Geometry: final body of the model. Coordinates: model frame, mm. A direction names the side the tool comes from. Round coordinates to 2 decimals unless told otherwise and drop trailing zeros. Loops run counter-clockwise (first coordinate to the right, second up) from the corner with the lowest first, then second, coordinate; pieces in that order, holes last. Notation, with made-up numbers: (-3, 50) - (14, 50) arc R11 cw to (14, 65) - close; hole circle Ø1 at (14, 39.25). An arc over 180 degrees is marked (long way). Return JSON: item names as keys, results as strings. Group by question number.
1. Section C-C on y = 20. Return loops of the section in (x, z) (3 decimals), and give its area (3 significant figures).
2. Section D-D on x = 88. Return loops of the section in (y, z) (3 decimals).
3. Section B-B on y = -39. Return loops of the section in (x, z) (3 decimals), and give its area (3 significant figures).
4. First-contact query: pin 1 Ø4 at (x, z) = (32, 19) entering from +Y; pin 2 Ø8 at (y, z) = (-10, 40) entering from +X; pin 3 Ø12 at (y, z) = (1, 50.5) entering from +X (3 decimals); pin 4 Ø15 at (y, z) = (-22.5, 19.5) entering from +X (3 decimals). Flat tips, straight axial feed; report the tip coordinate or a pass-through.
5. Material intervals for probe 1 along Y at (x, z) = (11, 39) (3 decimals); probe 2 along Z at (x, y) = (-19.5, 52) (3 decimals); probe 3 along X at (y, z) = (-22, 13) (3 decimals), sorted ascending.
6. Set-up query: faces 1 (the face through (32.73, -20.7, 51.97)), 2 (the face through (9, 0, 31)), 3 (the face through (45.8, -0.4, 38.1)), 4 (the face through (86, 0, 38.1)), 5 (the face through (47, -25.4, 42)). Return all of +Z, -Z, +X, -X, +Y, -Y with unobstructed straight access to the full face (end or side cutting, diameter ignored); none if empty.
7. Section A-A on z = 0. Return loops of the section in (x, y) (3 decimals).
from build123d import *

# Parameters (mm, degrees)
F1_DEPTH = 63.5
F0_W     = 25.7705491662
F0_H     = 19.05
F2_DEPTH = 25.4
F3_DEPTH = 15.875
F4_DEPTH = 25.4
F6_R     = 6.35


with BuildPart() as f1:
    # F0 (on Front) → F1 (new body, symmetric)
    with BuildSketch(Plane.XZ):
        Polygon((22.225, 9.525), (-41.275, 9.525), (-41.275, -9.525), (41.275, -9.525), (41.275, 9.525), align=None)
    extrude(amount=F1_DEPTH, both=True)

    # F0 (on Front) → F2 (join, symmetric)
    with BuildSketch(Plane.XZ):
        with BuildLine():
            Line((22.225, 27.0002), (22.225, 9.525))
            Line((22.225, 9.525), (41.275, 9.525))
            Line((41.275, 9.525), (41.275, 27.0002))
            ThreePointArc((41.275, 27.0002), (45.9246798487, 38.2255201513), (57.15, 42.8752))
            Line((57.15, 42.8752), (60.325, 42.8752))
            Line((60.325, 42.8752), (60.325, 61.9252))
            Line((60.325, 61.9252), (57.15, 61.9252))
            ThreePointArc((57.15, 61.9252), (32.4542956671, 51.6959043329), (22.225, 27.0002))
        make_face()
        with Locations((73.2102745831, 52.4002)):
            Rectangle(F0_W, F0_H)
    extrude(amount=F2_DEPTH, both=True)

    # F0 (on Front) → F3 (join)
    with BuildSketch(Plane.XZ):
        with BuildLine():
            add(Edge.make_bspline(
                [(-41.275, 9.525), (-11.6340629756, 43.7753386796), (15.0888795033, 63.8811737299), (57.15, 61.9252)],
                knots=[0, 0, 0, 0, 111.5045361635, 111.5045361635, 111.5045361635, 111.5045361635], degree=3))
            Line((-41.275, 9.525), (22.225, 9.525))
            Line((22.225, 9.525), (22.225, 27.0002))
            ThreePointArc((22.225, 27.0002), (32.4542956671, 51.6959043329), (57.15, 61.9252))
        make_face()
    extrude(amount=F3_DEPTH)

    # F0 (on Front) → F4 (join, symmetric)
    with BuildSketch(Plane.XZ):
        with Locations((73.2102745831, 52.4002)):
            Rectangle(F0_W, F0_H)
    extrude(amount=F4_DEPTH, both=True)

    # F0 (on Front) → F5 (revolve)
    with BuildSketch(Plane.XZ):
        Polygon((86.0955491662, 66.675), (86.0955491662, 61.9252), (86.0955491662, 42.8752), (86.0955491662, 38.1), (111.125, 38.1), (111.125, 66.675), align=None)
    revolve(axis=Axis((86.0955491662, 0, 52.3875), (0, 0, -1)))

    # F6
    f6_edges = [f1.edges().sort_by_distance(p)[0] for p in [
        (41.275, -63.5, 0),
        (-41.275, -63.5, 0),
        (-41.275, 0, -9.525),
        (0, 63.5, -9.525),
        (41.275, 0, -9.525),
        (0, -63.5, -9.525),
        (-41.275, 63.5, 0),
        (41.275, 63.5, 0),
    ]]
    fillet(f6_edges, radius=F6_R)


solid = f1.part
Taken from the geometry:
{
 "1": {"outline": "(-41.275, -3.175) arc R6.35 ccw to (-34.925, -9.525) - (34.925, -9.525) arc R6.35 ccw to (41.275, -3.175) - (41.275, 27) arc R15.875 cw to (57.15, 42.875) - (71.047, 42.875) - (71.047, 38.1) - (101.145, 38.1) - (101.145, 66.675) - (71.047, 66.675) - (71.047, 61.925) - (57.15, 61.925) arc R34.925 ccw to (22.225, 27) - (22.225, 9.525) - (-41.275, 9.525) - close", "area": "3,770 mm2"},
 "2": {"outline": "(-24.957, 38.1) - (24.957, 38.1) - (24.957, 66.675) - (-24.957, 66.675) - close"},
 "3": {"outline": "(-41.275, -3.175) arc R6.35 ccw to (-34.925, -9.525) - (34.925, -9.525) arc R6.35 ccw to (41.275, -3.175) - (41.275, 9.525) - (-41.275, 9.525) - close", "area": "1,560 mm2"},
 "4": {"pin 1": "y = 25.4", "pin 2": "x = 110.4", "pin 3": "x = 111.125", "pin 4": "x = 41.275"},
 "5": {"probe 1": "-15.875 to 0", "probe 2": "-9.525 to 9.525", "probe 3": "22.225 to 41.275"},
 "6": {"face 1": "+Z, -X, -Y", "face 2": "+Z, -X, +Y", "face 3": "-Z, +Y, -Y", "face 4": "-Z, +X, +Y, -Y", "face 5": "+Z, +X, -X, -Y"},
 "7": {"outline": "(-41.275, -57.15) arc R6.35 ccw to (-34.925, -63.5) - (34.925, -63.5) arc R6.35 ccw to (41.275, -57.15) - (41.275, 57.15) arc R6.35 ccw to (34.925, 63.5) - (-34.925, 63.5) arc R6.35 ccw to (-41.275, 57.15) - close"}
}
